Geometry check sheet. Reference: the model listing, model coordinates, mm. A direction names the side the tool comes from. Give positions to 0.01 mm unless a question says otherwise; leave off trailing zeros. Loops run counter-clockwise (first coordinate to the right, second up) from the corner with the lowest first, then second, coordinate; pieces in that order, holes last. Notation, with made-up numbers: (23, 71.5) -> (71, 71.5) arc R25 ccw to (71, 110.5) -> close; hole circle Ø5 at (-13.75, -8.5). An arc over 180 degrees is marked (long way). Answer as a JSON object with one key per item and string values.
from build123d import *

# Parameters (mm, degrees)
ESQUISSE1_W             = 7
ESQUISSE1_H             = 40
BOSS_EXTRU_1_DEPTH      = 5
ENL_V_MAT_EXTRU_1_DEPTH = 5
ESQUISSE3_W             = 3
ESQUISSE3_H             = 40
BOSS_EXTRU_2_DEPTH      = 6
ESQUISSE5_W             = 3
ESQUISSE5_H             = 10
BOSS_EXTRU_3_DEPTH      = 25
ESQUISSE4_R             = 1.625
ENL_V_MAT_EXTRU_2_DEPTH = 4
ESQUISSE9_W             = 3
ESQUISSE9_H             = 30
BOSS_EXTRU_5_DEPTH      = 25
ESQUISSE10_W            = 3
ESQUISSE10_H            = 15
BOSS_EXTRU_6_DEPTH      = 10
ESQUISSE11_W            = 10
ESQUISSE11_H            = 20
BOSS_EXTRU_7_DEPTH      = 17
ESQUISSE12_R            = 2.6
ENL_V_MAT_EXTRU_3_DEPTH = 5


with BuildPart() as part:
    # Esquisse1 → Boss.-Extru.1 (new body)
    with BuildSketch(Plane.XY):
        with Locations((3.5, -20)):
            Rectangle(ESQUISSE1_W, ESQUISSE1_H)
    extrude(amount=BOSS_EXTRU_1_DEPTH)

    # Esquisse2 → Enlèv. mat.-Extru.1 (cut)
    with BuildSketch(Plane.XY.offset(5)):
        Polygon((0, -40), (0, 0), (1.5, -40), align=None)
    extrude(amount=-ENL_V_MAT_EXTRU_1_DEPTH, mode=Mode.SUBTRACT)

    # Esquisse3 → Boss.-Extru.2 (add)
    with BuildSketch(Plane.XY.offset(5)):
        with Locations((5.5, -20)):
            Rectangle(ESQUISSE3_W, ESQUISSE3_H)
    extrude(amount=BOSS_EXTRU_2_DEPTH)

    # Esquisse5 → Boss.-Extru.3 (add)
    with BuildSketch(Plane.XY.offset(11)):
        with Locations((5.5, -5)):
            Rectangle(ESQUISSE5_W, ESQUISSE5_H)
    extrude(amount=BOSS_EXTRU_3_DEPTH)

    # Esquisse4 → Enlèv. mat.-Extru.2 (cut, through all)
    with BuildSketch(Plane.ZY.offset(-4)):
        with Locations((7.320815767, -35)):
            Circle(ESQUISSE4_R)
        with Locations((7.320815767, -5)):
            Circle(ESQUISSE4_R)
    extrude(amount=-ENL_V_MAT_EXTRU_2_DEPTH, mode=Mode.SUBTRACT)

    # Esquisse9 → Boss.-Extru.5 (add)
    with BuildSketch(Plane.XY.offset(11)):
        with Locations((5.5, -25)):
            Rectangle(ESQUISSE9_W, ESQUISSE9_H)
    extrude(amount=BOSS_EXTRU_5_DEPTH)

    # Esquisse10 → Boss.-Extru.6 (add)
    with BuildSketch(Plane.XZ.offset(40)):
        with Locations((5.5, 28.5)):
            Rectangle(ESQUISSE10_W, ESQUISSE10_H)
    extrude(amount=BOSS_EXTRU_6_DEPTH)

    # Esquisse11 → Boss.-Extru.7 (add)
    with BuildSketch(Plane.ZY.offset(-4)):
        with Locations((26, -40)):
            Rectangle(ESQUISSE11_W, ESQUISSE11_H)
    extrude(amount=BOSS_EXTRU_7_DEPTH)

    # Esquisse12 → Enlèv. mat.-Extru.3 (cut)
    with BuildSketch(Plane(origin=(0, 0, 21), x_dir=(-1, 0, 0), z_dir=(0, 0, -1))):
        with Locations((5.3, -44.1)):
            Circle(ESQUISSE12_R)
    extrude(amount=-ENL_V_MAT_EXTRU_3_DEPTH, mode=Mode.SUBTRACT)


solid = part.part
1) Tool access check on faces 1 (the face through (-3.384, -42.343, 23.465)), 2 (the face through (-4, -40, 31)), 3 (the face through (0.74, -19.72, 2.54)), 4 (the face through (5, -40, 8)). Record the directions out of +Z, -Z, +X, -X, +Y, -Y that give a thin tool (end or side, any length) a straight path to the whole face; none if there is none.
Geometry check:
{"face 1": "-Z", "face 2": "+Z, -X, +Y, -Y", "face 3": "-Z, -X, -Y", "face 4": "-Z, +X, -X, -Y"}
2) Section check A-A on x = -5.3. Record the cut outline in (y, z), plus the area to 3 significant figures.
Geometry check:
{"outline": "(-50, 21) -> (-46.7, 21) -> (-46.7, 26) -> (-41.5, 26) -> (-41.5, 21) -> (-30, 21) -> (-30, 31) -> (-50, 31) -> close", "area": "174 mm2"}
3) Material ranges on line 1 along Y through (x, z) = (-5.3, 22.05); line 2 along Z through (x, y) = (2.75, -14); line 3 along X through (y, z) = (-9, 9.5), recorded low to high. Write a range as from..to.
Geometry check:
{"line 1": "y = -50..-46.7, -41.5..-30", "line 2": "z = 0..5", "line 3": "x = 4..7"}
4) Section check B-B on z = 23. Record the cut outline in (x, y), plus the area to 3 significant figures.
Geometry check:
{"outline": "(-13, -50) -> (7, -50) -> (7, 0) -> (4, 0) -> (4, -30) -> (-13, -30) -> close; hole circle Ø5.2 at (-5.3, -44.1)", "area": "469 mm2"}
5) Depth check by flat-ended pin: P1, Ø5.5, axis at x = -6.5, y = -45, coming from the -Z side; P2, Ø3, axis at y = -25, z = 21, coming from the -X side; P3, Ø4.5, axis at x = 5.5, z = 12.5, coming from the -Y side. Enter the tip coordinate at first touch or a pass-through.
Geometry check:
{"P1": "stops at z = 21", "P2": "stops at x = 4", "P3": "stops at y = -40"}
6) Section check C-C on y = -44.1. Record the cut outline in (x, z), plus the area to 3 significant figures.
Geometry check:
{"outline": "(-13, 21) -> (-7.9, 21) -> (-7.9, 26) -> (-2.7, 26) -> (-2.7, 21) -> (7, 21) -> (7, 36) -> (4, 36) -> (4, 31) -> (-13, 31) -> close", "area": "189 mm2"}
7) Draft check along Z on faces 5 (the face through (5.48, -35.99, 6.03)), 6 (the face through (-4, -30, 26)), 7 (the face through (3, -20, 0)). Enter one of: pulls with the +Z half, pulls with the -Z half, needs draft (parallel to the pull), parting line crosses it, or undercut.
Geometry check:
{"face 5": "undercut", "face 6": "needs draft", "face 7": "pulls with the -Z half"}
8) Section check D-D on z = 7. Record the cut outline in (x, y), plus the area to 3 significant figures.
Geometry check:
{"outline": "(4, -40) -> (7, -40) -> (7, -36.59) -> (4, -36.59) -> close; (4, -33.41) -> (7, -33.41) -> (7, -6.59) -> (4, -6.59) -> close; (4, -3.41) -> (7, -3.41) -> (7, 0) -> (4, 0) -> close", "area": "101 mm2"}
